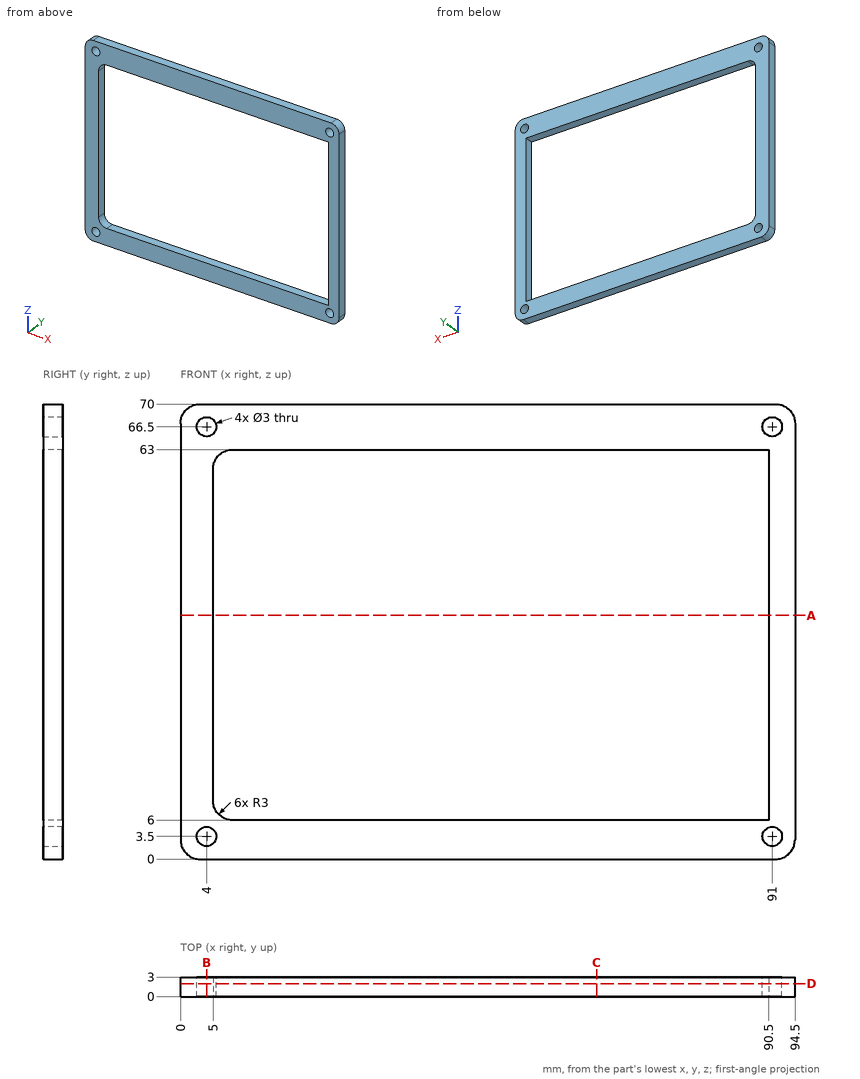
The figure shows three views and two pictorial views of one solid part (mm, origin at its lowest corner). Answer the questions. Round coordinates to 2 decimals unless told otherwise and drop trailing zeros. Write each loop counter-clockwise with the first axis right and the second up, starting at its lowest first coordinate (ties: lowest second). Pieces come first, ordered by that corner, then holes. Notation, with made-up numbers: (54, 70.25) - (112, 70.25) arc R7 ccw to (112, 81.25) - close; hole circle Ø5 at (26.5, 85.5). An arc over 180 degrees is marked (long way). Answer in a Markdown table with one row per item. Add a question column.
1. A cutting plane is placed at A-A, the plane z = 37.5. Determine the outline of the cut face in (x, y), and give its area (3 significant figures).
2. Given pin 1 (2.5 mm diameter, centred on x = 91, z = 3.5, fed in from +Y), flat-ended and moving along its own axis, determine where the tip first touches the part or whether it passes through.
3. Find the intervals of material crossed by line 1 along Z through (x, y) = (91, 0.95); line 2 along X through (y, z) = (1.55, 66.5); line 3 along Z through (x, y) = (24.5, 1.85), in increasing order. Write a range as from..to.
4. A cutting plane is placed at C-C, the plane x = 64. Determine the outline of the cut face in (y, z), and give its area (3 significant figures).
5. A cutting plane is placed at B-B, the plane x = 4. Determine the outline of the cut face in (y, z).
6. A cutting plane is placed at D-D, the plane y = 2. Determine the outline of the cut face in (x, z).
Worked out:
| question | item | result |
|---|---|---|
| 1 | outline | (0, 0) - (5, 0) - (5, 3) - (0, 3) - close; (90.5, 0) - (94.5, 0) - (94.5, 3) - (90.5, 3) - close |
| 1 | area | 27.0 mm^2 |
| 2 | pin 1 | through |
| 3 | line 1 | 0..2, 5..65, 68..70 |
| 3 | line 2 | 0..2.5, 5.5..89.5, 92.5..94.5 |
| 3 | line 3 | 0..6, 63..70 |
| 4 | outline | (0, 0) - (3, 0) - (3, 6) - (0, 6) - close; (0, 63) - (3, 63) - (3, 70) - (0, 70) - close |
| 4 | area | 39.0 mm^2 |
| 5 | outline | (0, 0) - (3, 0) - (3, 2) - (0, 2) - close; (0, 5) - (3, 5) - (3, 65) - (0, 65) - close; (0, 68) - (3, 68) - (3, 70) - (0, 70) - close |
| 6 | outline | (0, 3) arc R3 ccw to (3, 0) - (91.5, 0) arc R3 ccw to (94.5, 3) - (94.5, 67) arc R3 ccw to (91.5, 70) - (3, 70) arc R3 ccw to (0, 67) - close; hole circle Ø3 at (4, 3.5); hole circle Ø3 at (4, 66.5); hole (5, 9) arc R3 ccw to (8, 6) - (90.5, 6) - (90.5, 63) - (8, 63) arc R3 ccw to (5, 60) - close; hole circle Ø3 at (91, 3.5); hole circle Ø3 at (91, 66.5) |
